Verification items for the finished model (mm, model axes). A direction names the side the tool comes from. Give positions to 0.01 mm unless a question says otherwise; leave off trailing zeros. Order: outer loops, then holes, each group sorted by start corner. A loop starts at its lowest first (then second) coordinate and runs counter-clockwise, first axis right, second up. Notation, with made-up numbers: (-26, -22) -> (13, -22) arc R20 cw to (13, 14) -> close; hole circle Ø8 at (0, 37.5). An arc over 180 degrees is marked (long way). One line per question, with ' | ' between items. Start each with the question number.
Q1. Mould release check, pull along Y, two halves, no side actions. Record for faces 1 (the cylindrical face through (25.5, 4.31, 4.3)), 2 (the flat face through (0, -16, 6)), 3 (the flat face through (26, 0, 3)): released by +Y, released by -Y, zero draft, split by the parting line, or undercut.
Q2. Go/stop test with flat-tipped pins: pin 1 (0.8 mm diameter, centred on x = 25.5, z = 6.5, fed in from +Y) (3 decimals); pin 2 (5 mm diameter, centred on x = 7, y = 5.5, fed in from +Z). Record where each tip stops, or that it passes through.
Q3. Access from +Z, -Z, +X, -X, +Y, -Y to the whole of each face (thin tool, end or side, straight path). Record for faces 4 (the cylindrical face through (25.699, 15.715, 5.916)), 5 (the flat face through (-25.004, 0, 7)), 6 (the cylindrical face through (25.5, -5.12, 8.7)), 7 (the flat face through (0, 16, 6)), 8 (the flat face through (-25, 12, 1)).
Q4. Material ranges on probe 1 along X at (y, z) = (-8.5, 8); probe 2 along Y at (x, z) = (-5, 10.5); probe 3 along Z at (x, y) = (23.5, 6.5), recorded low to high. Write a range as [from, to].
Q5. Section check C-C on y = 0.5. Record the cut outline in (x, z).
Q6. Section check D-D on z = 9.75. Record the cut outline in (x, y), plus the area to 3 significant figures.
Q7. Section check B-B on z = 5.75. Record the cut outline in (x, y).
Q8. Section check A-A on x = 20.5. Record the cut outline in (y, z), plus the area to 3 significant figures.
from build123d import *

# Parameters (mm, degrees)
SKETCH1_W           = 52
SKETCH1_H           = 32
SKETCH1_W_2         = 50
SKETCH1_H_2         = 2.5
BOSS_EXTRUDE1_DEPTH = 2
SKETCH2_W           = 52
SKETCH2_H           = 32
SKETCH2_W_2         = 50.00793432
SKETCH2_H_2         = 30
BOSS_EXTRUDE2_DEPTH = 10
SKETCH3_W           = 5
SKETCH3_H           = 10
CUT_EXTRUDE1_DEPTH  = 10
FILLET1_R           = 1
FILLET2_R           = 1
FILLET3_R           = 1
FILLET4_R           = 1
FILLET5_R           = 1
FILLET6_R           = 1
FILLET7_R           = 1
FILLET8_R           = 1


with BuildPart() as part:
    # Sketch1 → Boss-Extrude1 (new body)
    with BuildSketch(Plane.XY):
        Rectangle(SKETCH1_W, SKETCH1_H)
        with Locations((0, 12.5)):
            Rectangle(SKETCH1_W_2, SKETCH1_H_2, mode=Mode.SUBTRACT)
        with Locations((0, -12.5)):
            Rectangle(SKETCH1_W_2, SKETCH1_H_2, mode=Mode.SUBTRACT)
    extrude(amount=BOSS_EXTRUDE1_DEPTH)

    # Sketch2 → Boss-Extrude2 (add)
    with BuildSketch(Plane.XY.offset(2)):
        Rectangle(SKETCH2_W, SKETCH2_H)
        Rectangle(SKETCH2_W_2, SKETCH2_H_2, mode=Mode.SUBTRACT)
    extrude(amount=BOSS_EXTRUDE2_DEPTH)

    # Sketch3 → Cut-Extrude1 (cut)
    with BuildSketch(Plane(origin=(26, 0, 0), x_dir=(0, 0, -1), z_dir=(1, 0, 0))):
        with Locations((-6.5, -0.40632889)):
            Rectangle(SKETCH3_W, SKETCH3_H)
    extrude(amount=-CUT_EXTRUDE1_DEPTH, mode=Mode.SUBTRACT)

    # Fillet1
    fillet1_edges = [part.edges().sort_by_distance(p)[0] for p in [
        (26, 16, 6),
    ]]
    fillet(fillet1_edges, radius=FILLET1_R)

    # Fillet2
    fillet2_edges = [part.edges().sort_by_distance(p)[0] for p in [
        (26, -16, 6),
    ]]
    fillet(fillet2_edges, radius=FILLET2_R)

    # Fillet3
    fillet3_edges = [part.edges().sort_by_distance(p)[0] for p in [
        (-26, -16, 6),
    ]]
    fillet(fillet3_edges, radius=FILLET3_R)

    # Fillet4
    fillet4_edges = [part.edges().sort_by_distance(p)[0] for p in [
        (-26, 16, 6),
    ]]
    fillet(fillet4_edges, radius=FILLET4_R)

    # Fillet5
    fillet5_edges = [part.edges().sort_by_distance(p)[0] for p in [
        (25.50198358, 4.59367111, 4),
    ]]
    fillet(fillet5_edges, radius=FILLET5_R)

    # Fillet6
    fillet6_edges = [part.edges().sort_by_distance(p)[0] for p in [
        (25.50198358, -5.40632889, 4),
    ]]
    fillet(fillet6_edges, radius=FILLET6_R)

    # Fillet7
    fillet7_edges = [part.edges().sort_by_distance(p)[0] for p in [
        (25.50198358, -5.40632889, 9),
    ]]
    fillet(fillet7_edges, radius=FILLET7_R)

    # Fillet8
    fillet8_edges = [part.edges().sort_by_distance(p)[0] for p in [
        (25.50198358, 4.59367111, 9),
    ]]
    fillet(fillet8_edges, radius=FILLET8_R)


solid = part.part
Filled in:
1) face 1: undercut | face 2: released by -Y | face 3: zero draft
2) pin 1: y = 15.995 | pin 2: z = 2
3) face 4: +Z, -Z, +X, +Y | face 5: +Z | face 6: +X | face 7: +Z, -Z, +X, -X, +Y | face 8: +Z, -Z
4) probe 1: [-26, -25], [25, 26] | probe 2: [-16, -15], [15, 16] | probe 3: [0, 2]
5) outline: (-26, 0) -> (26, 0) -> (26, 4) -> (25, 4) -> (25, 2) -> (-25, 2) -> (-25, 12) -> (-26, 12) -> close; (25, 9) -> (26, 9) -> (26, 12) -> (25, 12) -> close
6) outline: (-26, -15) arc R1 ccw to (-25, -16) -> (25, -16) arc R1 ccw to (26, -15) -> (26, 15) arc R1 ccw to (25, 16) -> (-25, 16) arc R1 ccw to (-26, 15) -> close; hole (-25, -15) -> (25, -15) -> (25, 15) -> (-25, 15) -> close | area: 163 mm²
7) outline: (-26, -15) arc R1 ccw to (-25, -16) -> (25, -16) arc R1 ccw to (26, -15) -> (26, -5.41) -> (25, -5.41) -> (25, -15) -> (-25, -15) -> (-25, 15) -> (25, 15) -> (25, 4.59) -> (26, 4.59) -> (26, 15) arc R1 ccw to (25, 16) -> (-25, 16) arc R1 ccw to (-26, 15) -> close
8) outline: (-16, 0) -> (-13.75, 0) -> (-13.75, 2) -> (-15, 2) -> (-15, 12) -> (-16, 12) -> close; (-11.25, 0) -> (11.25, 0) -> (11.25, 2) -> (-11.25, 2) -> close; (13.75, 0) -> (16, 0) -> (16, 12) -> (15, 12) -> (15, 2) -> (13.75, 2) -> close | area: 74.0 mm²
